Input: dimensioned drawing with shaded views. Units: mm. Origin: part minimum x, y, z. A direction names the side the tool comes from. Give positions to 0.01 mm unless a question says otherwise; leave off trailing zeros. Loops run counter-clockwise (first coordinate to the right, second up) from the corner with the lowest first, then second, coordinate; pieces in that order, holes last. Notation, with made-up numbers: (-36, 1) -> (-11, 1) arc R9 cw to (-11, 18) -> close; hole circle Ø5 at (13, 71). An arc over 180 degrees is marked (long way). Answer in a Markdown table with one row per item. Add a question column.
1) Section query B-B (y = 189). Return the cut outline in (x, z).
2) Section query A-A (y = 27.5). Return the cut outline in (x, z).
3) Section query D-D (z = 92). Return the cut outline in (x, y).
4) First-contact query: P1, Ø24, axis at x = 95.5, z = 67, coming from the +Y side. Flat tip, straight axial feed; report the tip coordinate or a pass-through.
5) Access query for the marked faces 1 and 2. Directions: +Z, -Z, +X, -X, +Y, -Y. A direction counts if a zero-diameter tool reaches every point of the face in a straight line with its end or side. Return the directions, or none.
6) Draft query along X for the marked faces 3, 4 and 5. Return one class per face: +X half, -X half, draft (parallel to the pull), parting line (faces both ways), or undercut.
7) Line query: line 1 (Z direction, x = 46.5, y = 150); line 2 (Y direction, x = 207.5, z = 66.5); line 3 (Y direction, x = 101, z = 112). Output: solid intervals per line, ascending. Write a range as from..to.
8) Section query C-C (x = 107). Return the cut outline in (y, z), plus the area to 3 significant figures.
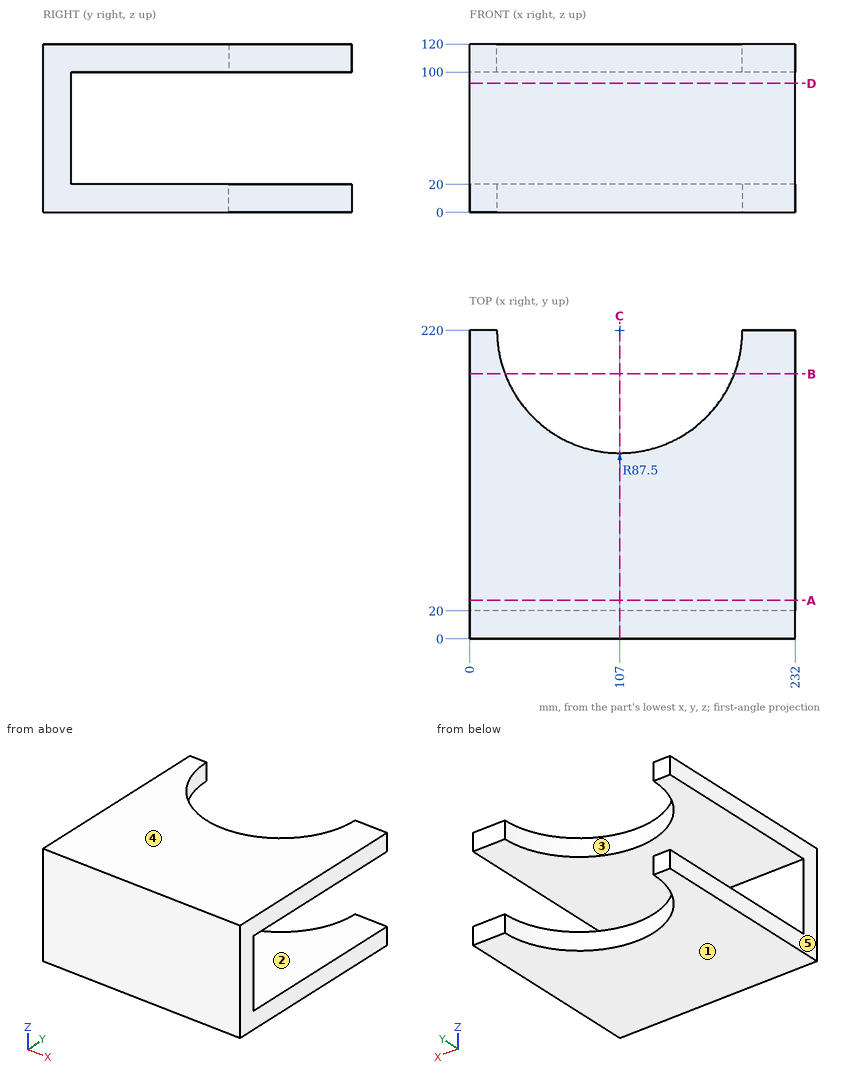
Evaluation:
| question | item | result |
|---|---|---|
| 1 | outline | (0, 0) -> (25.18, 0) -> (25.18, 20) -> (0, 20) -> close; (0, 100) -> (25.18, 100) -> (25.18, 120) -> (0, 120) -> close; (188.82, 0) -> (232, 0) -> (232, 20) -> (188.82, 20) -> close; (188.82, 100) -> (232, 100) -> (232, 120) -> (188.82, 120) -> close |
| 2 | outline | (0, 0) -> (232, 0) -> (232, 20) -> (0, 20) -> close; (0, 100) -> (232, 100) -> (232, 120) -> (0, 120) -> close |
| 3 | outline | (0, 0) -> (232, 0) -> (232, 20) -> (0, 20) -> close |
| 4 | P1 | y = 20 |
| 5 | face 1 | -Z, +X, -X, +Y, -Y |
| 5 | face 2 | +X, -X, +Y |
| 6 | face 3 | undercut |
| 6 | face 4 | draft |
| 6 | face 5 | -X half |
| 7 | line 1 | 0..20, 100..120 |
| 7 | line 2 | 0..20 |
| 7 | line 3 | 0..132.71 |
| 8 | outline | (0, 0) -> (132.5, 0) -> (132.5, 20) -> (20, 20) -> (20, 100) -> (132.5, 100) -> (132.5, 120) -> (0, 120) -> close |
| 8 | area | 6,900 mm² |
